For this review, take the finished solid that the model builds, in its own axes (mm). A direction names the side the tool comes from. Coordinates: 2 decimals unless noted, no trailing zeros. Loops run counter-clockwise (first coordinate to the right, second up) from the corner with the lowest first, then second, coordinate; pieces in that order, holes last. Notation, with made-up numbers: (66.25, 78.25) - (96.25, 78.25) arc R21 cw to (96.25, 100.25) - close; hole circle Ø3 at (66.5, 78.5). An arc over 180 degrees is marked (long way). Use one line per item in the form item = value. Start each with the question number.
1. Add section C-C on x = -1.5. Give the boundary of the cut face in (y, z), and give its area (3 significant figures).
2. Machinability: for faces 1 (the face through (2.71, -0.37, -1.66)), 2 (the face through (-0.25, 0.723, -1.081)), which of the approach directions +Z, -Z, +X, -X, +Y, -Y give a long, thin tool a straight path to every point of the face, cutting with its end or side? Answer none if there is none.
3. For pin 1 Ø1.5 at (x, y) = (-2.5, -0.5) entering from +Z; pin 2 Ø2 at (y, z) = (1, 0.5) entering from +X, all flat-tipped, find the tip position at first contact; note any pin that passes through.
4. Add section B-B on z = 2. Count the separate pieces of the cut face and the enclosed holes in it, and give its area (3 significant figures).
5. To check wall thickness, follow probe 1 along Y at (x, z) = (0, 0); probe 2 along Z at (x, y) = (-2.25, 0); probe 3 along Z at (x, y) = (2, -0.5). State the ranges of each line that lie inside material, in increasing order.
6. Add section A-A on x = -2.5. Give the boundary of the cut face in (y, z).
7. Draft analysis for pull direction X (two halves, no side actions). For faces 3 (the face through (3.4, -0.4, -1.4)), 4 (the face through (-2.7, -0.37, -1.66)), state which applies: +X half, -X half, draft (parallel to the pull), parting line (faces both ways), or undercut.
Autodesk Inventor part; units mm, degrees
ref_plane "Plano de trabajo2" through (2.75, 0, 0) normal (1, 0, 0) x (0, 1, 0)
ref_plane "Plano de trabajo3" through (-2.75, 0, 0) normal (1, 0, 0) x (0, 1, 0)
ref_plane "Plano de trabajo6" through (2.75, 0, 0) normal (1, 0, 0) x (0, 1, 0)
sketch "Boceto1" plane through (0, 0, 0) normal (0, 0, 1) x (1, 0, 0)
  arc A0 (0, -2.75) -> (0, 2.75) centre (0, 0) ccw
  line L0 (0, 2.75) -> (0, -2.75)
  dimension "d0" = 5.5
revolve "Revolución1" add sketch "Boceto1" angle 360 about axis through (0, 2.75, 0) along (0, -1, 0)
ref_plane "Plano de trabajo2" through (2.75, 0, 0) normal (1, 0, 0) x (0, 1, 0)
ref_plane "Plano de trabajo3" through (-2.75, 0, 0) normal (1, 0, 0) x (0, 1, 0)
sketch "Boceto7" plane through (2.75, 0, 0) normal (1, 0, 0) x (0, 1, 0)
  circle A0 centre (0, 0) radius 1.7
  circle A1 centre (0, 0) radius 1.3
  dimension "d21" = 3.4
  dimension "d22" = 0.4
extrude "Extrusión5" add sketch "Boceto7" along normal blind 0.5 and the other way blind 1
sketch "Boceto8" plane through (-2.75, 0, 0) normal (1, 0, 0) x (0, 1, 0)
  circle A0 centre (0, 0) radius 1.7
  circle A1 centre (0, 0) radius 1.7
  circle A2 centre (0, 0) radius 1.3
  dimension "d27" = 3.4
  dimension "d35" = 2.6
extrude "Extrusión6" add sketch "Boceto8" along normal blind 1 and the other way blind 0.5 contours A0 | A2
ref_plane "Plano de trabajo6" through (2.75, 0, 0) normal (1, 0, 0) x (0, 1, 0)
sketch "Boceto10" plane through (2.75, 0, 0) normal (1, 0, 0) x (0, 1, 0)
  circle A0 centre (0, 0) radius 1.3
extrude "Extrusión8" cut sketch "Boceto10" against normal blind 10
ref_plane "Plano de trabajo7" through (3.25, 0, 0) normal (1, 0, 0) x (0, 0, -1)
sketch "Boceto11" plane through (3.25, 0, 0) normal (1, 0, 0) x (0, 0, -1)
  circle A0 centre (0, 0) radius 2.1
  circle A1 centre (0, 0) radius 1.3
  dimension "d39" = 4.2
extrude "Extrusión9" add sketch "Boceto11" along normal blind 0.15
ref_plane "Plano de trabajo9" through (-3.7, 0, 0) normal (-1, 0, 0) x (0, 0, 1)
ref_plane "Plano de trabajo8" through (-3.25, 0, 0) normal (-1, 0, 0) x (0, 0, 1)
sketch "Boceto12" plane through (-3.7, 0, 0) normal (-1, 0, 0) x (0, 0, 1)
  circle A0 centre (0, 0) radius 3.03
  circle A1 centre (0, 0) radius 1.3
  dimension "d44" = 6.06
extrude "Extrusión10" add sketch "Boceto12" along normal blind 0.1 and the other way blind 0.45
fillet "Empalme1" radius 2 1 edges at (-3.25, 0, -3.03)
properties part number "Bola grande" material "Aluminio 6061"
Conclusion:
q1.outline = circle Ø4.61 at (0, 0); hole circle Ø2.6 at (0, 0)
q1.area = 11.4 mm^2
q2.face_1 = none
q2.face_2 = +X, -X
q3.pin_1 = 2.08
q3.pin_2 = 3.4
q4.separate_pieces = 3
q4.enclosed_holes = 0
q4.area = 13.1 mm^2
q5.probe_1 = -2.75 to -1.3, 1.3 to 2.75
q5.probe_2 = -1.7 to -1.3, 1.3 to 1.7
q5.probe_3 = -1.82 to -1.2, 1.2 to 1.82
q6.outline = circle Ø3.4 at (0, 0); hole circle Ø2.6 at (0, 0)
q7.face_3 = +X half
q7.face_4 = undercut
